Model file for the job. Use its own axes, mm. A direction names the side the tool comes from. Coordinates: 2 decimals unless noted, no trailing zeros. Write each loop counter-clockwise with the first axis right and the second up, starting at its lowest first coordinate (ties: lowest second). Pieces come first, ordered by that corner, then holes. Notation, with made-up numbers: M -39.75,62 L -29.75,62 A20 cw -29.75,96 Z; hole C -23,23 d11. An arc over 180 degrees is marked long. One line per question, with ' | ' between items. Start each with the question number.
(1) Wall check: probe 1 along Y at (x, z) = (8.5, 0.45); probe 2 along Z at (x, y) = (-1, -4). Give the ranges that are in metal, low to high.
(2) Cut at A-A (x = 8.5). Write the cut outline in (y, z).
(3) Flat gauge pins, fed straight in: pin 1 Ø1 at (x, z) = (-6.5, 2.5) entering from +Y; pin 2 Ø2.5 at (x, y) = (-8.5, 8.5) entering from -Z; pin 3 Ø2.5 at (x, y) = (-8.5, -8.5) entering from +Z; pin 4 Ø0.8 at (y, z) = (0.5, 2.5) entering from -X. Where does each tip first touch, or does it go through?
(4) Cut at C-C (y = 1.75). Write the cut outline in (x, z).
(5) Tool access for faces 1 (the face through (-1.85, 0, 2)), 2 (the face through (11.5, 0, 1)), 3 (the face through (0, 2.5, 2)): list every direction of +Z, -Z, +X, -X, +Y, -Y with a clear straight run to the whole face (end or side of a thin tool).
(6) Two-plate mould, pull along X, no slides. Class faces 4 (the face through (0, -2.5, 2)), 5 (the face through (-8.37, -9.49, 0.76)), 6 (the face through (8.63, 7.51, 0.76)), 7 (the face through (1.85, 0, 2)): +X half, -X half, draft (parallel to the pull), parting line (faces both ways), or undercut.
(7) Cut at D-D (z = 1.15). Write the cut outline in (x, y).
Autodesk Fusion 360 part; units mm, degrees
sketch "Sketch1" plane through (0, 0, 0) normal (0, 0, 1) x (1, 0, 0)
  line L0 (11.5, 11.5) -> (-11.5, 11.5)
  line L1 (-11.5, 11.5) -> (-11.5, -11.5)
  line L2 (-11.5, -11.5) -> (11.5, -11.5)
  line L3 (11.5, -11.5) -> (11.5, 11.5)
  line L4 (11.5, 11.5) -> (-11.5, -11.5) construction
  line L5 (-11.5, 11.5) -> (11.5, -11.5) construction
  dimension "d1" = 23
  dimension "d2" = 23
extrude "Extrude1" add sketch "Sketch1" along normal blind 1.5
chamfer "Chamfer1" distance 1 angle 45 4 edges at (-11.5, -11.5, 0.75) (11.5, -11.5, 0.75) (11.5, 11.5, 0.75) (-11.5, 11.5, 0.75)
sketch "Sketch2" plane through (0, 0, 1.5) normal (0, 0, 1) x (-1, 0, 0)
  line L0 (10.5, -11.5) -> (11.5, -10.5)
  line L1 (11.5, -10.5) -> (11.5, 10.5)
  line L2 (11.5, 10.5) -> (10.5, 11.5)
  line L3 (10.5, 11.5) -> (-10.5, 11.5)
  line L4 (-10.5, 11.5) -> (-11.5, 10.5)
  line L5 (-11.5, 10.5) -> (-11.5, -10.5)
  line L6 (-11.5, -10.5) -> (-10.5, -11.5)
  line L7 (-10.5, -11.5) -> (10.5, -11.5)
  line L8 (-1.85, 2.5) -> (1.85, 2.5)
  line L9 (1.85, 2.5) -> (1.85, -2.5)
  line L10 (1.85, -2.5) -> (-1.85, -2.5)
  line L11 (-1.85, -2.5) -> (-1.85, 2.5)
  line L12 (-1.85, 2.5) -> (1.85, -2.5) construction
  line L13 (1.85, 2.5) -> (-1.85, -2.5) construction
  dimension "d6" = 3.7
  dimension "d7" = 5
extrude "Extrude2" add sketch "Sketch2" along normal blind 1.7 contours L8 L9 L10 L11
sketch "Sketch3" plane through (0, 0, 1.5) normal (0, 0, 1) x (-1, 0, 0)
  line L0 (-1.85, -2.5) -> (-1.85, 2.5)
  line L1 (-1.85, 2.5) -> (1.85, 2.5)
  line L2 (1.85, 2.5) -> (1.85, -2.5)
  line L3 (1.85, -2.5) -> (-1.85, -2.5)
  line L4 (10.5, -11.5) -> (11.5, -10.5)
  line L5 (11.5, -10.5) -> (11.5, 10.5)
  line L6 (11.5, 10.5) -> (10.5, 11.5)
  line L7 (10.5, 11.5) -> (-10.5, 11.5)
  line L8 (-10.5, 11.5) -> (-11.5, 10.5)
  line L9 (-11.5, 10.5) -> (-11.5, -10.5)
  line L10 (-11.5, -10.5) -> (-10.5, -11.5)
  line L11 (-10.5, -11.5) -> (10.5, -11.5)
  line L12 (-8.5, -8.5) -> (8.5, -8.5) construction
  line L13 (8.5, -8.5) -> (8.5, 8.5) construction
  line L14 (8.5, 8.5) -> (-8.5, 8.5) construction
  line L15 (-8.5, 8.5) -> (-8.5, -8.5) construction
  line L16 (-8.5, -8.5) -> (8.5, 8.5) construction
  line L17 (8.5, -8.5) -> (-8.5, 8.5) construction
  circle A0 centre (8.5, -8.5) radius 1
  circle A1 centre (-8.5, -8.5) radius 1
  circle A2 centre (-8.5, 8.5) radius 1
  circle A3 centre (8.5, 8.5) radius 1
  dimension "d10" = 2
  dimension "d11" = 17
extrude "Extrude3" cut sketch "Sketch3" against normal up to surface (1.5 mm away) contours A0 | A1 | A2 | A3
equation "d8 = 3.2 mm - 1.5 mm"
Filled in:
1) probe 1: -11.5 to -9.5, -7.5 to 7.5, 9.5 to 11.5 | probe 2: 0 to 1.5
2) outline: M -11.5,0 L -9.5,0 L -9.5,1.5 L -11.5,1.5 Z; M -7.5,0 L 7.5,0 L 7.5,1.5 L -7.5,1.5 Z; M 9.5,0 L 11.5,0 L 11.5,1.5 L 9.5,1.5 Z
3) pin 1: through | pin 2: z = 0 | pin 3: z = 1.5 | pin 4: x = -1.85
4) outline: M -11.5,0 L 11.5,0 L 11.5,1.5 L 1.85,1.5 L 1.85,3.2 L -1.85,3.2 L -1.85,1.5 L -11.5,1.5 Z
5) face 1: +Z, -X, +Y, -Y | face 2: +Z, -Z, +X, +Y, -Y | face 3: +Z, +X, -X, +Y
6) face 4: draft | face 5: undercut | face 6: undercut | face 7: +X half
7) outline: M -11.5,-10.5 L -10.5,-11.5 L 10.5,-11.5 L 11.5,-10.5 L 11.5,10.5 L 10.5,11.5 L -10.5,11.5 L -11.5,10.5 Z; hole C -8.5,-8.5 d2; hole C -8.5,8.5 d2; hole C 8.5,-8.5 d2; hole C 8.5,8.5 d2
